```python
from build123d import *

# Parameters (mm, degrees)
SKETCH_1_W               = 25
SKETCH_1_H               = 25
SKETCH_1_W_2             = 19
SKETCH_1_H_2             = 19
EXTRUDE_1_DEPTH          = 350
SKETCH_2_R               = 3
CUT_EXTRUDE_1_DEPTH      = 352.781181987
CUT_EXTRUDE_2_DEPTH      = 352.781181987
CUT_EXTRUDE_2_DEPTH_BACK = 352.781181987
SKETCH_3_R               = 1.5


with BuildPart() as part:
    # 草图1 → 凸台-拉伸1 (new body)
    with BuildSketch(Plane(origin=(0, 0, 0), x_dir=(1, 0, 0), z_dir=(0, 1, 0))):
        with Locations((12.5, 12.5)):
            Rectangle(SKETCH_1_W, SKETCH_1_H)
        with Locations((12.5, 12.5)):
            Rectangle(SKETCH_1_W_2, SKETCH_1_H_2, mode=Mode.SUBTRACT)
    extrude(amount=EXTRUDE_1_DEPTH)

    # 草图2 → 切除-拉伸1 (cut, through all)
    with BuildSketch(Plane(origin=(0, 0, 0), x_dir=(0, 0, -1), z_dir=(1, 0, 0))):
        with Locations(Location((12.5, 10, 0), (0, 0, 180))):
            Circle(SKETCH_2_R)
        with Locations(Location((12.5, 40, 0), (0, 0, 180))):
            Circle(SKETCH_2_R)
        with Locations(Location((12.5, 70, 0), (0, 0, 180))):
            Circle(SKETCH_2_R)
    extrude(amount=CUT_EXTRUDE_1_DEPTH, mode=Mode.SUBTRACT)

    # 草图3 → 切除-拉伸2 (cut, two sides: drawn at the far end of the back side and taken through both)
    with BuildSketch(Plane.XY.offset(-CUT_EXTRUDE_2_DEPTH_BACK)):
        with Locations((6, 250)):
            Circle(SKETCH_3_R)
        with Locations((6, 285)):
            Circle(SKETCH_3_R)
    extrude(amount=CUT_EXTRUDE_2_DEPTH + CUT_EXTRUDE_2_DEPTH_BACK, mode=Mode.SUBTRACT)


solid = part.part
```
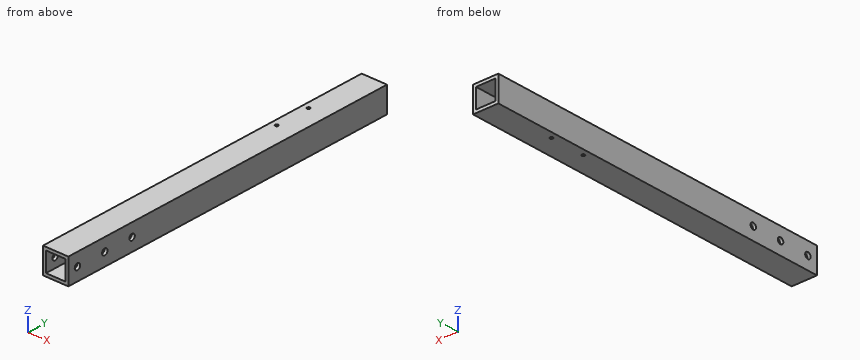
Work out the finished part from the listing and answer in its coordinate system (mm). Give positions to 0.01 mm unless a question says otherwise; leave off trailing zeros. Loops run counter-clockwise (first coordinate to the right, second up) from the corner with the lowest first, then second, coordinate; pieces in that order, holes last. Notation, with made-up numbers: (39.5, 65.5) - (85.5, 65.5) arc R23 cw to (85.5, 83.5) - close; hole circle Ø6 at (33, 20.25). An arc over 180 degrees is marked (long way). Use CSV: the item, a comma, the result in double quotes. Start each with the question number.
(1) Find the intervals of material crossed by L1, parallel to Y at x = 23.6, z = -12.5; L2, parallel to Y at x = 6, z = -23; L3, parallel to X at y = 117.5, z = -13, in increasing order.
(2) This flat-tipped pin is pushed along its axis until it touches: pin 1 (5 mm diameter, centred on y = 40, z = -12.5, fed in from +X). Where does it stop, or does it pass through?
(3) Find section A-A, the plane y = 10. Determine the outline of the cut face in (x, z), plus the area to 3 significant figures.
(4) Find section B-B, the plane x = 13. Determine the outline of the cut face in (y, z).
(5) Find section C-C, the plane y = 183.5. Determine the outline of the cut face in (x, z), plus the area to 3 significant figures.
(6) Find section D-D, the plane z = -12.5. Count the separate pieces of the cut face and the enclosed holes in it, plus the area to 3 significant figures.
Results found:
1,L1,"0 to 7, 13 to 37, 43 to 67, 73 to 350"
1,L2,"0 to 248.5, 251.5 to 283.5, 286.5 to 350"
1,L3,"0 to 3, 22 to 25"
2,pin 1,"through"
3,outline,"(0, -25) - (25, -25) - (25, -15.5) - (22, -15.5) - (22, -22) - (3, -22) - (3, -15.5) - (0, -15.5) - close; (0, -9.5) - (3, -9.5) - (3, -3) - (22, -3) - (22, -9.5) - (25, -9.5) - (25, 0) - (0, 0) - close"
3,area,"228 mm^2"
4,outline,"(0, -25) - (350, -25) - (350, -22) - (0, -22) - close; (0, -3) - (350, -3) - (350, 0) - (0, 0) - close"
5,outline,"(0, -25) - (25, -25) - (25, 0) - (0, 0) - close; hole (3, -22) - (22, -22) - (22, -3) - (3, -3) - close"
5,area,"264 mm^2"
6,separate pieces,"8"
6,enclosed holes,"0"
6,area,"1,990 mm^2"
